Work out the finished part from the listing and answer in its coordinate system (mm). A direction names the side the tool comes from. Give positions to 0.01 mm unless a question says otherwise; leave off trailing zeros. Loops run counter-clockwise (first coordinate to the right, second up) from the corner with the lowest first, then second, coordinate; pieces in that order, holes last. Notation, with made-up numbers: (3.25, 18.25) - (31.25, 18.25) arc R24 ccw to (31.25, 34.25) - close; hole circle Ø1 at (69.25, 71). An arc over 180 degrees is marked (long way). One line per question, with ' | ' between items. Start each with the question number.
1. Section C-C (x = -6) is taken. Determine the outline of the cut face in (y, z), plus the area to 3 significant figures.
2. Find the intervals of material crossed by line 1 (X direction, y = 7.5, z = -6.5); line 2 (Y direction, x = 7.5, z = -4); line 3 (Y direction, x = -8.5, z = 5.75), in increasing order.
3. Which of the six approach directions +Z, -Z, +X, -X, +Y, -Y give full straight-line access (tool end or side, diameter ignored) to faces 5 (the face through (-8, 7, 0)), 6 (the face through (22, 12.5, 0))?
4. Each of these flat-tipped pins is pushed along its axis until it touches: pin 1 (5 mm diameter, centred on x = -3.5, y = 3.5, fed in from -Z); pin 2 (4.5 mm diameter, centred on x = -2.5, z = 1.5, fed in from +Y). Where does it stop, or does it pass through?
5. Section B-B (z = 0.75) is taken. Determine the outline of the cut face in (x, y), plus the area to 3 significant figures.
6. For a pull along X with two mould halves and no side action, classify faces 1 (the face through (8, 7, 0)), 2 (the face through (35, 0, 0)), 3 (the face through (-35, 0, 0)), 4 (the face through (0, -1, 7.75)) as released by +X, released by -X, zero draft, split by the parting line, or undercut.
7. Section A-A (y = 4.75) is taken. Determine the outline of the cut face in (x, z).
from build123d import *

# Parameters (mm, degrees)
SKETCH1_W           = 15.5
SKETCH1_H           = 25
BOSS_EXTRUDE1_DEPTH = 35
SKETCH2_W           = 16
SKETCH2_H           = 18.5
CUT_EXTRUDE1_DEPTH  = 16.5
FILLET1_R           = 1
FILLET2_R           = 1


with BuildPart() as part:
    # Sketch1 → Boss-Extrude1 (new body, symmetric)
    with BuildSketch(Plane(origin=(0, 0, 0), x_dir=(0, 0, -1), z_dir=(1, 0, 0))):
        Rectangle(SKETCH1_W, SKETCH1_H)
    extrude(amount=BOSS_EXTRUDE1_DEPTH, both=True)

    # Sketch2 → Cut-Extrude1 (cut, through all)
    with BuildSketch(Plane.XY.offset(7.75)):
        with Locations((0, 12.5)):
            Rectangle(SKETCH2_W, SKETCH2_H)
    extrude(amount=-CUT_EXTRUDE1_DEPTH, mode=Mode.SUBTRACT)

    # Fillet1
    fillet1_edges = [part.edges().sort_by_distance(p)[0] for p in [
        (8, 12.5, 0),
        (-8, 12.5, 0),
    ]]
    fillet(fillet1_edges, radius=FILLET1_R)

    # Fillet2
    fillet2_edges = [part.edges().sort_by_distance(p)[0] for p in [
        (-8, 7.375, 7.75),
        (8, 7.375, 7.75),
        (8, 7.375, -7.75),
        (-22, 12.5, 7.75),
        (-8.292893219, 12.207106781, 7.75),
        (8.292893219, 12.207106781, 7.75),
        (-22, 12.5, -7.75),
        (-8, 7.375, -7.75),
        (-8.292893219, 12.207106781, -7.75),
        (8.292893219, 12.207106781, -7.75),
        (22, 12.5, 7.75),
        (22, 12.5, -7.75),
    ]]
    fillet(fillet2_edges, radius=FILLET2_R)


solid = part.part
Conclusion:
1) outline: (-12.5, -7.75) - (3.25, -7.75) - (3.25, 7.75) - (-12.5, 7.75) - close | area: 244 mm²
2) line 1: -35 to -8, 8 to 35 | line 2: -12.5 to 3.25 | line 3: -12.5 to 12.37
3) face 5: +Z, -Z, +Y | face 6: +Z, -Z, +X, -X, +Y
4) pin 1: z = -7.75 | pin 2: y = 3.25
5) outline: (-35, -12.5) - (35, -12.5) - (35, 12.5) - (9, 12.5) arc R1 ccw to (8, 11.5) - (8, 3.25) - (-8, 3.25) - (-8, 11.5) arc R1 ccw to (-9, 12.5) - (-35, 12.5) - close | area: 1,600 mm²
6) face 1: undercut | face 2: released by +X | face 3: released by -X | face 4: zero draft
7) outline: (-35, -7.75) - (-9, -7.75) arc R1 ccw to (-8, -6.75) - (-8, 6.75) arc R1 ccw to (-9, 7.75) - (-35, 7.75) - close; (8, -6.75) arc R1 ccw to (9, -7.75) - (35, -7.75) - (35, 7.75) - (9, 7.75) arc R1 ccw to (8, 6.75) - close
